from build123d import *

# Parameters (mm, degrees)
SKETCH_1_W                   = 87.6
SKETCH_1_H                   = 140
EXTRUDE_1_DEPTH              = 12
CHAMFER_1_SIZE               = 5
HOLE_WIZARD_M6_1_D           = 6.6
HOLE_WIZARD_M6_1_CBORE_D     = 11
HOLE_WIZARD_M6_1_CBORE_DEPTH = 6
SKETCH_4_R                   = 2
CUT_EXTRUDE_1_DEPTH          = 84.441236808
SKETCH_5_R                   = 3.25
CUT_EXTRUDE_2_DEPTH          = 84.441236808


with BuildPart() as part:
    # 草图1 → 凸台-拉伸1 (new body)
    with BuildSketch(Plane.XY):
        Rectangle(SKETCH_1_W, SKETCH_1_H)
    extrude(amount=EXTRUDE_1_DEPTH)

    # 倒角1
    chamfer_1_edges = [part.edges().sort_by_distance(p)[0] for p in [
        (43.8, -70, 6),
        (-43.8, -70, 6),
        (-43.8, 70, 6),
        (43.8, 70, 6),
    ]]
    chamfer(chamfer_1_edges, length=CHAMFER_1_SIZE)

    # M6 六角凹头螺钉的柱形沉头孔1 (through all)
    with Locations(Plane.XY.offset(12)):
        with Locations((33.8, 50), (0, 50), (-33.8, 50), (-33.8, -50), (0, -50), (33.8, -50)):
            CounterBoreHole(HOLE_WIZARD_M6_1_D / 2, HOLE_WIZARD_M6_1_CBORE_D / 2, HOLE_WIZARD_M6_1_CBORE_DEPTH)

    # 草图4 → 切除-拉伸1 (cut, through all)
    with BuildSketch(Plane.XY.offset(12)):
        with Locations((-23.8, 57)):
            Circle(SKETCH_4_R)
        with Locations((23.8, 57)):
            Circle(SKETCH_4_R)
        with Locations((23.8, -43)):
            Circle(SKETCH_4_R)
        with Locations((-23.8, -43)):
            Circle(SKETCH_4_R)
    extrude(amount=-CUT_EXTRUDE_1_DEPTH, mode=Mode.SUBTRACT)

    # 草图5 → 切除-拉伸2 (cut, through all)
    with BuildSketch(Plane(origin=(0, 0, 0), x_dir=(-1, 0, 0), z_dir=(0, 0, -1))):
        with Locations((33.8, 62.5)):
            Circle(SKETCH_5_R)
        with Locations((0, 62.5)):
            Circle(SKETCH_5_R)
        with Locations((-33.8, 62.5)):
            Circle(SKETCH_5_R)
        with Locations((33.8, -62.5)):
            Circle(SKETCH_5_R)
        with Locations((0, -62.5)):
            Circle(SKETCH_5_R)
        with Locations((-33.8, -62.5)):
            Circle(SKETCH_5_R)
    extrude(amount=-CUT_EXTRUDE_2_DEPTH, mode=Mode.SUBTRACT)


solid = part.part
Build history of the part. All positions in model axes, mm. A direction names the side the tool comes from. Coordinates: 2 decimals unless noted, no trailing zeros. Write each loop counter-clockwise with the first axis right and the second up, starting at its lowest first coordinate (ties: lowest second). Pieces come first, ordered by that corner, then holes.
(1) 3-axis set-ups, long thin cutter, end or side, ignore diameter. For faces 1 (the cylindrical face through (-33.377, -59.278, 5.916)), 2 (the flat face through (-30, -50, 6)): which of +Z, -Z, +X, -X, +Y, -Y reach the whole face in a straight line?
(2) Mould opens along Y. For faces 3 (the flat face through (-41.3, -67.5, 5.9)), 4 (the cylindrical face through (2.395, 64.697, 5.916)), 5 (the flat face through (-43.8, -1, 6)) say: pulls with the +Y half, pulls with the -Y half, needs draft (parallel to the pull), parting line crosses it, or undercut.
(3) Cut at C-C on z = 1.5. State how many separate pieces and enclosed holes the cut face has, and give its area (3 significant figures).
(4) Cut at D-D on x = -23.8. List the corners of the cut face in (y, z), and give its area (3 significant figures).
(5) Cut at A-A on y = 50. List the corners of the cut face in (x, z).
(6) Pin check, flat tips, straight feed: pin 1 Ø6 at (x, y) = (0, 62.5) entering from -Z; pin 2 Ø10.5 at (x, y) = (0, 50) entering from +Z. Stop position of each tip, or through.
(7) Cut at B-B on x = 33.8. List the corners of the cut face in (y, z), and give its area (3 significant figures).
(8) Drill centre lines: line 1 (X direction, y = -49.5, z = 2.75); line 2 (Y direction, x = 0, z = 4.6); line 3 (Y direction, x = 33.8, z = 6.5). Where is each one in solid material? Low to high.
Working result:
1. face 1: +Z, -Z
1. face 2: +Z
2. face 3: pulls with the -Y half
2. face 4: undercut
2. face 5: needs draft
3. separate pieces: 1
3. enclosed holes: 16
3. area: 11,800 mm2
4. outline: (-70, 0) - (-45, 0) - (-45, 12) - (-70, 12) - close; (-41, 0) - (55, 0) - (55, 12) - (-41, 12) - close; (59, 0) - (70, 0) - (70, 12) - (59, 12) - close
4. area: 1,580 mm2
5. outline: (-43.8, 0) - (-37.1, 0) - (-37.1, 6) - (-39.3, 6) - (-39.3, 12) - (-43.8, 12) - close; (-30.5, 0) - (-3.3, 0) - (-3.3, 6) - (-5.5, 6) - (-5.5, 12) - (-28.3, 12) - (-28.3, 6) - (-30.5, 6) - close; (3.3, 0) - (30.5, 0) - (30.5, 6) - (28.3, 6) - (28.3, 12) - (5.5, 12) - (5.5, 6) - (3.3, 6) - close; (37.1, 0) - (43.8, 0) - (43.8, 12) - (39.3, 12) - (39.3, 6) - (37.1, 6) - close
6. pin 1: passes through
6. pin 2: stops at z = 6
7. outline: (-70, 0) - (-65.75, 0) - (-65.75, 12) - (-70, 12) - close; (-59.25, 0) - (-53.3, 0) - (-53.3, 6) - (-55.5, 6) - (-55.5, 12) - (-59.25, 12) - close; (-46.7, 0) - (46.7, 0) - (46.7, 6) - (44.5, 6) - (44.5, 12) - (-44.5, 12) - (-44.5, 6) - (-46.7, 6) - close; (53.3, 0) - (59.25, 0) - (59.25, 12) - (55.5, 12) - (55.5, 6) - (53.3, 6) - close; (65.75, 0) - (70, 0) - (70, 12) - (65.75, 12) - close
7. area: 1,310 mm2
8. line 1: x = -43.8 to -37.06, -30.54 to -3.26, 3.26 to 30.54, 37.06 to 43.8
8. line 2: y = -70 to -65.75, -59.25 to -53.3, -46.7 to 46.7, 53.3 to 59.25, 65.75 to 70
8. line 3: y = -70 to -65.75, -59.25 to -55.5, -44.5 to 44.5, 55.5 to 59.25, 65.75 to 70
